For this review, take the finished solid that the model builds, in its own axes (mm). A direction names the side the tool comes from. Coordinates: 2 decimals unless noted, no trailing zeros. Order: outer loops, then holes, each group sorted by start corner. A loop starts at its lowest first (then second) coordinate and runs counter-clockwise, first axis right, second up. Notation, with made-up numbers: (75.5, 69) - (95.5, 69) arc R15 ccw to (95.5, 85) - close; hole circle Ø3 at (75, 21.5). An arc over 180 degrees is marked (long way). One line per item, written item: value. Start each with the question number.
(1) To check wall thickness, follow line 1 along Y through (x, z) = (-0.5, 2.55); line 2 along Z through (x, y) = (-2.25, 7); line 3 along X through (y, z) = (4.5, 1.1). State the ranges of each line that lie inside material, in increasing order.
(2) Consider section A-A on z = 1.5. Write out the cut boundary in (x, y).
(3) Consider section B-B on x = 0.75. Write out the cut boundary in (y, z).
(4) Clearance check with flat-ended pins moving along their axes: pin 1 (1 mm diameter, centred on x = -2.5, z = 2.5, fed in from +Y); pin 2 (2 mm diameter, centred on x = 0, y = 6.5, fed in from +Z); pin 3 (1 mm diameter, centred on x = -1.5, y = -3.5, fed in from -Z). State where each tip first meets the part, or that it passes through.
(5) For faces 1 (the flat face through (0, 1, 0)), 2 (the flat face through (0, 7, 0.45)), list the 3-axis set-ups (+Z, -Z, +X, -X, +Y, -Y) from which the entire face can be reached by the end or side of a thin tool; tool diameter is ignored.
(6) Consider section C-C on x = -3.25. Write out the cut boundary in (y, z).
Autodesk Inventor part; units mm, degrees
ref_plane "YZ Plane" through (0, 0, 0) normal (1, 0, 0) x (0, 1, 0)
ref_plane "XZ Plane" through (0, 0, 0) normal (0, 1, 0) x (-1, 0, 0)
ref_plane "XY Plane" through (0, 0, 0) normal (0, 0, 1) x (1, 0, 0)
sketch "スケッチ1" plane through (0, 0, 0) normal (0, 0, 1) x (1, 0, 0)
  line L0 (-5, -5) -> (5, -5)
  line L1 (5, -5) -> (5, 5)
  line L2 (5, 5) -> (-5, 5)
  line L3 (-5, 5) -> (-5, -5)
  line L4 (-5, -5) -> (5, 5) construction
  line L5 (5, -5) -> (-5, 5) construction
  point P0 (0, 0)
  dimension "d0" = 10
  dimension "d1" = 10
extrude "押し出し1" add sketch "スケッチ1" along normal blind 4.05
sketch "スケッチ2" plane through (-5, 5, 0) normal (0, 1, 0) x (1, 0, 0)
  line L0 (5, 0) -> (2.15, 0)
  line L1 (10, 0) -> (0, 0)
  line L2 (2.15, 0) -> (7.85, 0)
  line L3 (7.85, 0) -> (7.85, -0.45)
  line L4 (7.85, -0.45) -> (2.15, -0.45)
  line L5 (2.15, -0.45) -> (2.15, 0)
  dimension "d4" = 2.85
  dimension "d5" = 5.7
  dimension "d6" = 0.45
extrude "押し出し2" add sketch "スケッチ2" along normal blind 3.9
fillet "フィレット1" radius 1 4 edges at (5, 5, 2.025) (5, -5, 2.025) (-5, 5, 2.025) (-5, -5, 2.025)
properties part number "VLV101040A"
Geometry check:
1. line 1: y = -5 to 5
1. line 2: z = 0 to 0.45
1. line 3: x = -4.87 to 4.87
2. outline: (-5, -4) arc R1 ccw to (-4, -5) - (4, -5) arc R1 ccw to (5, -4) - (5, 4) arc R1 ccw to (4, 5) - (-4, 5) arc R1 ccw to (-5, 4) - close
3. outline: (-5, 0) - (8.9, 0) - (8.9, 0.45) - (5, 0.45) - (5, 4.05) - (-5, 4.05) - close
4. pin 1: stops at y = 5
4. pin 2: stops at z = 0.45
4. pin 3: stops at z = 0
5. face 1: -Z, +X, -X, +Y, -Y
5. face 2: +Z, +X, -X, +Y
6. outline: (-5, 0) - (5, 0) - (5, 4.05) - (-5, 4.05) - close
